Source: CAD feature listing. Evaluate the final solid. Frame: model axes, mm. A direction names the side the tool comes from. Coordinates: 2 decimals unless noted, no trailing zeros. Order: outer loops, then holes, each group sorted by start corner. A loop starts at its lowest first (then second) coordinate and runs counter-clockwise, first axis right, second up. Notation, with made-up numbers: (7, 78) - (25, 78) arc R10 ccw to (25, 85) - close; hole circle Ø8 at (62, -21.5). An arc over 180 degrees is marked (long way). One line per question, with ' | ' between items.
from build123d import *

# Parameters (mm, degrees)
CYLINDER067_R     = 1.6
CYLINDER067_DEPTH = 2
BOX164_W          = 17
BOX164_H          = 2
BOX164_DEPTH      = 11
FILLET036_R       = 5
BOX165_W          = 4
BOX165_H          = 2
BOX165_DEPTH      = 1.5
BOX167_W          = 4
BOX167_H          = 2
BOX167_DEPTH      = 1.5
BOX166_W          = 4
BOX166_H          = 2
BOX166_DEPTH      = 1.5
BOX168_W          = 4
BOX168_H          = 2
BOX168_DEPTH      = 1.5


with BuildPart() as cylinder148:
    # Cylinder067 → Cylinder067 (new body)
    with BuildSketch(Plane(origin=(46.5, -17, -9), x_dir=(1, 0, 0), z_dir=(0, -1, 0))):
        Circle(CYLINDER067_R)
    extrude(amount=CYLINDER067_DEPTH)


with BuildPart() as cut092:
    # Box164 → Box164 (new body)
    with BuildSketch(Plane(origin=(38, -19, -12), x_dir=(1, 0, 0), z_dir=(0, 0, 1))):
        with Locations((8.5, 1)):
            Rectangle(BOX164_W, BOX164_H)
    extrude(amount=BOX164_DEPTH)

    # Fillet036
    fillet036_edges = [cut092.edges().sort_by_distance(p)[0] for p in [
        (38, -18, -12),
        (55, -18, -12),
    ]]
    fillet(fillet036_edges, radius=FILLET036_R)

    # Cut092: cut Cylinder148
    add(cylinder148.part, mode=Mode.SUBTRACT)


with BuildPart() as cube154:
    # Box165 → Box165 (new body)
    with BuildSketch(Plane(origin=(39, -17, -2.5), x_dir=(1, 0, 0), z_dir=(0, 0, 1))):
        with Locations((2, 1)):
            Rectangle(BOX165_W, BOX165_H)
    extrude(amount=BOX165_DEPTH)


with BuildPart() as cube156:
    # Box167 → Box167 (new body)
    with BuildSketch(Plane(origin=(50, -17, -8), x_dir=(1, 0, 0), z_dir=(0, 0, 1))):
        with Locations((2, 1)):
            Rectangle(BOX167_W, BOX167_H)
    extrude(amount=BOX167_DEPTH)


with BuildPart() as cube155:
    # Box166 → Box166 (new body)
    with BuildSketch(Plane(origin=(39, -17, -8), x_dir=(1, 0, 0), z_dir=(0, 0, 1))):
        with Locations((2, 1)):
            Rectangle(BOX166_W, BOX166_H)
    extrude(amount=BOX166_DEPTH)


with BuildPart() as fusion052:
    # Box168 → Box168 (new body)
    with BuildSketch(Plane(origin=(50, -17, -2.5), x_dir=(1, 0, 0), z_dir=(0, 0, 1))):
        with Locations((2, 1)):
            Rectangle(BOX168_W, BOX168_H)
    extrude(amount=BOX168_DEPTH)

    # Fusion052: union Cut092, Cube154, Cube156, Cube155
    add(cut092.part)
    add(cube154.part)
    add(cube156.part)
    add(cube155.part)


solid = fusion052.part
(1) Set-up query: faces 4 (the flat face through (52, -16, -6.5)), 5 (the flat face through (54, -16, -2)), 6 (the flat face through (43, -16, -2)). Return all of +Z, -Z, +X, -X, +Y, -Y with unobstructed straight access to the full face (end or side cutting, diameter ignored); none if empty.
Taken from the geometry:
face 4: +X, -X, +Y | face 5: +Z, -Z, +X, +Y | face 6: +Z, -Z, +Y
(2) Cut plane B-B (x = 46.5). Return the cut outline in (y, z), and give its area (3 significant figures).
Taken from the geometry:
outline: (-19, -12) - (-17, -12) - (-17, -10.6) - (-19, -10.6) - close; (-19, -7.4) - (-17, -7.4) - (-17, -1) - (-19, -1) - close | area: 15.6 mm²
(3) Material intervals for L1, parallel to X at y = -16.95, z = -7.25; L2, parallel to Z at x = 40.5, y = -16.55; L3, parallel to Z at x = 46.5, y = -17.5, sorted ascending. Write a range as from..to.
Taken from the geometry:
L1: x = 39..43, 50..54 | L2: z = -8..-6.5, -2.5..-1 | L3: z = -12..-10.6, -7.4..-1
(4) Pin query (flat end, axial travel): P1, Ø1, axis at x = 41.5, y = -15.5, coming from the -Z side; P2, Ø3.5, axis at x = 46.5, z = -9, coming from the +Y side; P3, Ø1.2, axis at y = -16, z = -1.5, coming from the +X side. Return the tip coordinate at first contact, or that it passes through.
Taken from the geometry:
P1: stops at z = -8 | P2: stops at y = -17 | P3: stops at x = 54
(5) Cut plane D-D (y = -17.55). Return the cut outline in (x, z).
Taken from the geometry:
outline: (38, -7) arc R5 ccw to (43, -12) - (50, -12) arc R5 ccw to (55, -7) - (55, -1) - (38, -1) - close; hole circle Ø3.2 at (46.5, -9)
(6) Cut plane A-A (y = -15.9). Return the cut outline in (x, z), and give its area (3 significant figures).
Taken from the geometry:
outline: (39, -8) - (43, -8) - (43, -6.5) - (39, -6.5) - close; (39, -2.5) - (43, -2.5) - (43, -1) - (39, -1) - close; (50, -8) - (54, -8) - (54, -6.5) - (50, -6.5) - close; (50, -2.5) - (54, -2.5) - (54, -1) - (50, -1) - close | area: 24.0 mm²
(7) Pull-direction query (Z, two-part tool) for faces 1 (the flat face through (46, -18, -12)), 2 (the flat face through (38, -18, -4)), 3 (the flat face through (41, -16, -2.5)); classes: pulls with the +Z half, pulls with the -Z half, needs draft (parallel to the pull), parting line crosses it, or undercut.
Taken from the geometry:
face 1: pulls with the -Z half | face 2: needs draft | face 3: undercut
(8) Cut plane C-C (z = -9). Return the cut outline in (x, y).
Taken from the geometry:
outline: (38.42, -19) - (44.9, -19) - (44.9, -17) - (38.42, -17) - close; (48.1, -19) - (54.58, -19) - (54.58, -17) - (48.1, -17) - close
